Verification items for the finished model (mm, model axes). Face numbers are marked on the shaded views. A direction names the side the tool comes from. Coordinates: 2 decimals unless noted, no trailing zeros. One line per item, written item: value.
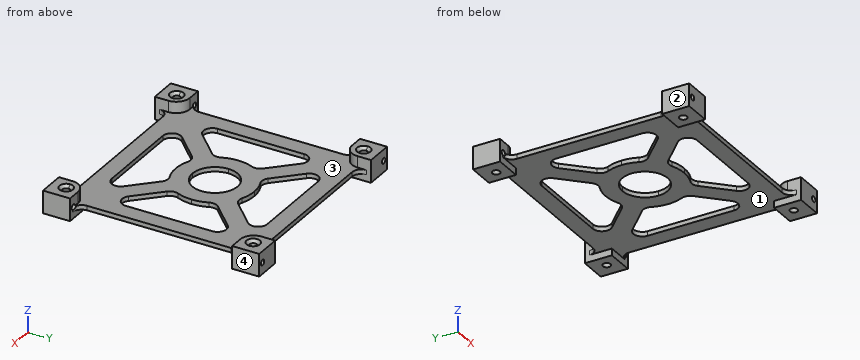
```python
from build123d import *

# Parameters (mm, degrees)
BOTTOMLAYER_DEPTH              = 10
BOSS_EXTRUDE1_DEPTH            = 2
M3_CLEARANCE_HOLE1_D           = 3.4
M3_CLEARANCE_HOLE1_CSINK_D     = 6
M3_CLEARANCE_HOLE1_CSINK_ANGLE = 90
TAP_DRILL_FOR_M3_TAP1_D        = 2.5
CIRPATTERN2_COUNT              = 4
CIRPATTERN3_OUTLINE_R          = 1.7
CIRPATTERN3_DEPTH              = 8.6999999
CIRPATTERN3_2_OUTLINE_W        = 12
CIRPATTERN3_2_OUTLINE_H        = 12
CIRPATTERN3_2_OUTLINE_R        = 1.7
CIRPATTERN3_2_DEPTH            = 8.6999999
CIRPATTERN3_START              = -48
CIRPATTERN3_3_OUTLINE_W        = 12
CIRPATTERN3_3_OUTLINE_H        = 1.3000001
CIRPATTERN3_3_DEPTH            = 12
CIRPATTERN3_START_2            = 36
CIRPATTERN3_4_OUTLINE_W        = 12
CIRPATTERN3_4_OUTLINE_H        = 1.3000001
CIRPATTERN3_4_DEPTH            = 12
FILLET1_R                      = 4
TAP_DRILL_FOR_M3_TAP2_D        = 2.5
TAP_DRILL_FOR_M3_TAP2_DEPTH    = 12
FILLET2_R                      = 4
FILLET3_R                      = 6


with BuildPart() as part:
    # Sketch3 → BottomLayer (new body)
    with BuildSketch(Plane.XY):
        Polygon((48, 48), (36, 48), (36, 42), (36, 36), (42, 36), (48, 36), align=None)
    extrude(amount=BOTTOMLAYER_DEPTH)

    # Sketch30 → Boss-Extrude1 (add)
    with BuildSketch(Plane.XY.offset(3)):
        with BuildLine():
            Line((0, 42), (42, 42))
            Line((42, 42), (42, 0))
            Line((42, 0), (34.5, 0))
            Line((34.5, 0), (34.5, 28.843145751))
            Line((34.5, 28.843145751), (14.875210928, 9.218356678))
            ThreePointArc((14.875210928, 9.218356678), (16.831015882, 4.792379824), (17.5, 0))
            Line((17.5, 0), (10, 0))
            ThreePointArc((10, 0), (7.071067812, 7.071067812), (0, 10))
            Line((0, 10), (0, 17.5))
            ThreePointArc((0, 17.5), (4.792379824, 16.831015882), (9.218356678, 14.875210928))
            Line((9.218356678, 14.875210928), (28.843145751, 34.5))
            Line((28.843145751, 34.5), (0, 34.5))
            Line((0, 34.5), (0, 42))
        make_face()
    boss_extrude1 = extrude(amount=BOSS_EXTRUDE1_DEPTH)

    # M3 Clearance Hole1 (through all)
    with Locations(Plane.XY.offset(10)):
        with Locations((41.525, 41.525)):
            CounterSinkHole(M3_CLEARANCE_HOLE1_D / 2, M3_CLEARANCE_HOLE1_CSINK_D / 2, counter_sink_angle=M3_CLEARANCE_HOLE1_CSINK_ANGLE)

    # Tap Drill for M3 Tap1 (through all)
    with Locations(Plane(origin=(0, 48, 0), x_dir=(1, 0, 0), z_dir=(0, 1, 0))):
        with Locations((45.5, -5)):
            tap_drill_for_m3_tap1 = Hole(TAP_DRILL_FOR_M3_TAP1_D / 2)

    # CirPattern2: Boss-Extrude1 ×4 about axis
    cirpattern2_axis = Axis((0, 0, 0), (0, 0, 1))
    for i in range(1, CIRPATTERN2_COUNT):
        add(boss_extrude1.rotate(cirpattern2_axis, i * 360 / CIRPATTERN2_COUNT))

    # CirPattern3: read off the stored shape, not the designer's step
    # CirPattern3 outline → CirPattern3 (cut)
    with BuildSketch(Plane.XY):
        with Locations((-41.525, 41.525)):
            Circle(CIRPATTERN3_OUTLINE_R)
        with Locations((-41.525, -41.525)):
            Circle(CIRPATTERN3_OUTLINE_R)
        with Locations((41.525, -41.525)):
            Circle(CIRPATTERN3_OUTLINE_R)
    extrude(amount=CIRPATTERN3_DEPTH, mode=Mode.SUBTRACT)

    # CirPattern3 2 outline → CirPattern3 2 (add)
    # profile 1 of 3: a face of its own
    with BuildSketch(Plane.XY):
        with Locations((-42, 42)):
            Rectangle(CIRPATTERN3_2_OUTLINE_W, CIRPATTERN3_2_OUTLINE_H)
        with Locations((-41.525, 41.525)):
            Circle(CIRPATTERN3_2_OUTLINE_R, mode=Mode.SUBTRACT)
    # profile 2 of 3: a face of its own
    with BuildSketch(Plane.XY):
        with Locations((42, -42)):
            Rectangle(CIRPATTERN3_2_OUTLINE_W, CIRPATTERN3_2_OUTLINE_H)
        with Locations((41.525, -41.525)):
            Circle(CIRPATTERN3_2_OUTLINE_R, mode=Mode.SUBTRACT)
    # profile 3 of 3: a face of its own
    with BuildSketch(Plane.XY):
        with Locations((-42, -42)):
            Rectangle(CIRPATTERN3_2_OUTLINE_W, CIRPATTERN3_2_OUTLINE_H)
        with Locations((-41.525, -41.525)):
            Circle(CIRPATTERN3_2_OUTLINE_R, mode=Mode.SUBTRACT)
    extrude(amount=CIRPATTERN3_2_DEPTH)

    # CirPattern3 3 outline → CirPattern3 3 (add)
    with BuildSketch(Plane(origin=(0, 0, 0), x_dir=(1, 0, 0), z_dir=(0, 1, 0)).offset(CIRPATTERN3_START)):
        with Locations((42, -9.34999995)):
            Rectangle(CIRPATTERN3_3_OUTLINE_W, CIRPATTERN3_3_OUTLINE_H)
        with Locations((-42, -9.34999995)):
            Rectangle(CIRPATTERN3_3_OUTLINE_W, CIRPATTERN3_3_OUTLINE_H)
    extrude(amount=CIRPATTERN3_3_DEPTH)

    # CirPattern3 4 outline → CirPattern3 4 (add)
    with BuildSketch(Plane(origin=(0, 0, 0), x_dir=(1, 0, 0), z_dir=(0, 1, 0)).offset(CIRPATTERN3_START_2)):
        with Locations((-42, -9.34999995)):
            Rectangle(CIRPATTERN3_4_OUTLINE_W, CIRPATTERN3_4_OUTLINE_H)
    extrude(amount=CIRPATTERN3_4_DEPTH)

    # CirPattern3 5: loft between two sections, ruled curve by curve
    cirpattern3_5_from = [
        Edge.make_three_point_arc((-39.825, 41.525, 8.7), (-41.525, 43.225, 8.7), (-43.225, 41.525, 8.7)),
        Edge.make_three_point_arc((-43.225, 41.525, 8.7), (-41.525, 39.825, 8.7), (-39.825, 41.525, 8.7)),
    ]
    cirpattern3_5_to = [
        Edge.make_three_point_arc((-38.525, 41.525, 10), (-41.525, 44.525, 10), (-44.525, 41.525, 10)),
        Edge.make_three_point_arc((-44.525, 41.525, 10), (-41.525, 38.525, 10), (-38.525, 41.525, 10)),
    ]
    cirpattern3_5 = Solid(Shell([*[Face.make_surface_from_curves(cirpattern3_5_from[k], cirpattern3_5_to[k]) for k in range(2)], Face(Wire(cirpattern3_5_from)), Face(Wire(cirpattern3_5_to))]))
    add(cirpattern3_5, mode=Mode.SUBTRACT)

    # CirPattern3 6: loft between two sections, ruled curve by curve
    cirpattern3_6_from = [
        Edge.make_three_point_arc((-39.825, -41.525, 8.7), (-41.525, -39.825, 8.7), (-43.225, -41.525, 8.7)),
        Edge.make_three_point_arc((-43.225, -41.525, 8.7), (-41.525, -43.225, 8.7), (-39.825, -41.525, 8.7)),
    ]
    cirpattern3_6_to = [
        Edge.make_three_point_arc((-38.525, -41.525, 10), (-41.525, -38.525, 10), (-44.525, -41.525, 10)),
        Edge.make_three_point_arc((-44.525, -41.525, 10), (-41.525, -44.525, 10), (-38.525, -41.525, 10)),
    ]
    cirpattern3_6 = Solid(Shell([*[Face.make_surface_from_curves(cirpattern3_6_from[k], cirpattern3_6_to[k]) for k in range(2)], Face(Wire(cirpattern3_6_from)), Face(Wire(cirpattern3_6_to))]))
    add(cirpattern3_6, mode=Mode.SUBTRACT)

    # CirPattern3 7: loft between two sections, ruled curve by curve
    cirpattern3_7_from = [
        Edge.make_three_point_arc((43.225, -41.525, 8.7), (41.525, -39.825, 8.7), (39.825, -41.525, 8.7)),
        Edge.make_three_point_arc((39.825, -41.525, 8.7), (41.525, -43.225, 8.7), (43.225, -41.525, 8.7)),
    ]
    cirpattern3_7_to = [
        Edge.make_three_point_arc((44.525, -41.525, 10), (41.525, -38.525, 10), (38.525, -41.525, 10)),
        Edge.make_three_point_arc((38.525, -41.525, 10), (41.525, -44.525, 10), (44.525, -41.525, 10)),
    ]
    cirpattern3_7 = Solid(Shell([*[Face.make_surface_from_curves(cirpattern3_7_from[k], cirpattern3_7_to[k]) for k in range(2)], Face(Wire(cirpattern3_7_from)), Face(Wire(cirpattern3_7_to))]))
    add(cirpattern3_7, mode=Mode.SUBTRACT)

    # Fillet1
    fillet1_edges = [part.edges().sort_by_distance(p)[0] for p in [
        (28.843145751, 34.5, 4),
        (9.218356678, 14.875210928, 4),
        (14.875210928, 9.218356678, 4),
        (34.5, 28.843145751, 4),
        (-34.5, -28.843145751, 4),
        (-34.5, 28.843145751, 4),
        (-14.875210928, 9.218356678, 4),
        (-9.218356678, 14.875210928, 4),
        (-28.843145751, 34.5, 4),
        (28.843145751, -34.5, 4),
        (-28.843145751, -34.5, 4),
        (-9.218356678, -14.875210928, 4),
        (-14.875210928, -9.218356678, 4),
        (34.5, -28.843145751, 4),
        (14.875210928, -9.218356678, 4),
        (9.218356678, -14.875210928, 4),
    ]]
    fillet(fillet1_edges, radius=FILLET1_R)

    # Tap Drill for M3 Tap2
    with Locations(Plane(origin=(0, 48, 0), x_dir=(1, 0, 0), z_dir=(0, 1, 0))):
        with Locations((-45.5, -5)):
            tap_drill_for_m3_tap2 = Hole(TAP_DRILL_FOR_M3_TAP2_D / 2, depth=TAP_DRILL_FOR_M3_TAP2_DEPTH)

    # Mirror1: Tap Drill for M3 Tap1, Tap Drill for M3 Tap2 across plane
    add(tap_drill_for_m3_tap1.mirror(Plane.ZX), mode=Mode.SUBTRACT)
    add(tap_drill_for_m3_tap2.mirror(Plane.ZX), mode=Mode.SUBTRACT)

    # Fillet2
    # the kernel refuses this fillet: 4 mm, written as the material it adds along each edge
    with BuildSketch(Plane(origin=(-42, 36, 5), x_dir=(-1, 0, 0), z_dir=(0, 0, -1))) as fillet2_piece_1_section:
        with BuildLine():
            CenterArc((FILLET2_R, -FILLET2_R), FILLET2_R, 90, 90)
            Line((0, -FILLET2_R), (0, 0))
            Line((0, 0), (FILLET2_R, 0))
        make_face()
    fillet2_piece_1 = extrude(amount=2, mode=Mode.PRIVATE)
    fillet2_piece_1 = fillet2_piece_1 - Plane(origin=(-45.5, 36, 5), x_dir=(-1, 0, 0), z_dir=(0, -1, 0)) * Cylinder(1.25, 20, mode=Mode.PRIVATE)
    add(fillet2_piece_1)
    with BuildSketch(Plane(origin=(-36, 42, 3), x_dir=(1, 0, 0), z_dir=(0, 0, 1)), Plane(origin=(-36, -42, 5), x_dir=(1, 0, 0), z_dir=(0, 0, -1)), Plane(origin=(36, -42, 3), x_dir=(-1, 0, 0), z_dir=(0, 0, 1))) as fillet2_piece_2:
        with BuildLine():
            CenterArc((FILLET2_R, FILLET2_R), FILLET2_R, 180, 90)
            Line((0, FILLET2_R), (0, 0))
            Line((0, 0), (FILLET2_R, 0))
        make_face()
    extrude(amount=2)
    with BuildSketch(Plane(origin=(-42, -36, 3), x_dir=(0, 1, 0), z_dir=(0, 0, 1))) as fillet2_piece_3_section:
        with BuildLine():
            CenterArc((FILLET2_R, FILLET2_R), FILLET2_R, 180, 90)
            Line((0, FILLET2_R), (0, 0))
            Line((0, 0), (FILLET2_R, 0))
        make_face()
    fillet2_piece_3 = extrude(amount=2, mode=Mode.PRIVATE)
    fillet2_piece_3 = fillet2_piece_3 - Plane(origin=(-45.5, -36, 5), x_dir=(-1, 0, 0), z_dir=(0, 1, 0)) * Cylinder(1.25, 20, mode=Mode.PRIVATE)
    add(fillet2_piece_3)
    with BuildSketch(Plane(origin=(42, -36, 5), x_dir=(1, 0, 0), z_dir=(0, 0, -1))) as fillet2_piece_4_section:
        with BuildLine():
            CenterArc((FILLET2_R, -FILLET2_R), FILLET2_R, 90, 90)
            Line((0, -FILLET2_R), (0, 0))
            Line((0, 0), (FILLET2_R, 0))
        make_face()
    fillet2_piece_4 = extrude(amount=2, mode=Mode.PRIVATE)
    fillet2_piece_4 = fillet2_piece_4 - Plane(origin=(45.5, -36, 5), x_dir=(-1, 0, 0), z_dir=(0, 1, 0)) * Cylinder(1.25, 20, mode=Mode.PRIVATE)
    add(fillet2_piece_4)
    with BuildSketch(Plane(origin=(42, 36, 5), x_dir=(0, -1, 0), z_dir=(0, 0, -1))) as fillet2_piece_5_section:
        with BuildLine():
            CenterArc((FILLET2_R, -FILLET2_R), FILLET2_R, 90, 90)
            Line((0, -FILLET2_R), (0, 0))
            Line((0, 0), (FILLET2_R, 0))
        make_face()
    fillet2_piece_5 = extrude(amount=2, mode=Mode.PRIVATE)
    fillet2_piece_5 = fillet2_piece_5 - Plane(origin=(45.5, 36, 5), x_dir=(-1, 0, 0), z_dir=(0, -1, 0)) * Cylinder(1.25, 20, mode=Mode.PRIVATE)
    add(fillet2_piece_5)
    with BuildSketch(Plane(origin=(36, 42, 3), x_dir=(-1, 0, 0), z_dir=(0, 0, 1))) as fillet2_piece_6:
        with BuildLine():
            CenterArc((FILLET2_R, -FILLET2_R), FILLET2_R, 90, 90)
            Line((0, -FILLET2_R), (0, 0))
            Line((0, 0), (FILLET2_R, 0))
        make_face()
    extrude(amount=2)

    # Fillet3
    fillet3_edges = [part.edges().sort_by_distance(p)[0] for p in [
        (36, 36, 7.5),
        (-36, 36, 7.5),
        (-36, -36, 7.5),
        (36, -36, 7.5),
    ]]
    fillet(fillet3_edges, radius=FILLET3_R - 0.0001)  # a hair under: the kernel refuses the full size


solid = part.part
```
Item 1: Draft check along Y on the marked faces 1 and 2. Enter one of: released by +Y, released by -Y, zero draft, split by the parting line, or undercut.
The answers:
face 1: undercut
face 2: zero draft
Item 2: Go/stop test with flat-tipped pins: P1, Ø4, axis at x = 45.5, z = 5, coming from the +Y side; P2, Ø0.6, axis at y = 2.5, z = 4.5, coming from the +X side; P3, Ø5.5, axis at x = -41.525, y = -41.525, coming from the +Z side; P4, Ø3, axis at x = -8.5, z = 4.5, coming from the -Y side. Record where each tip stops, or that it passes through.
The answers:
P1: stops at y = 48
P2: stops at x = 42
P3: stops at z = 9.75
P4: stops at y = -42
Item 3: Scan lines: line 1 (X direction, y = -20, z = 4.75); line 2 (Y direction, x = 11.5, z = 4); line 3 (Y direction, x = 13.5, z = 4.75). Record each from-to range of solid material in increasing order.
The answers:
line 1: x = -42 to -34.42, -25.66 to -14.34, 14.34 to 25.66, 34.42 to 42
line 2: y = -42 to -34.5, -17.16 to 17.16, 34.5 to 42
line 3: y = -42 to -34.5, -19.16 to 19.16, 34.5 to 42
Item 4: Access from +Z, -Z, +X, -X, +Y, -Y to the whole of each face (thin tool, end or side, straight path). Record for the marked faces 3 and 4.
The answers:
face 3: +Z
face 4: +Z, -Z, +X, +Y, -Y
